```python
from build123d import *

# Parameters (mm, degrees)
SKETCH1_R           = 51.308
BOSS_EXTRUDE1_DEPTH = 92.71
SKETCH2_W           = 103.886
SKETCH2_H           = 103.886
SKETCH2_R           = 1.27
BOSS_EXTRUDE2_DEPTH = 1.27
SHELL1_START        = -92.71
SHELL1_OUTLINE_R    = 50.038
SHELL1_DEPTH        = 92.71
FILLET1_R           = 12.7
SKETCH3_R           = 2.9591
BOSS_EXTRUDE3_DEPTH = 36.83


# Read off the part's stored shape, not the designer's step: Shell1
with BuildPart() as part:
    # Sketch1 → Boss-Extrude1 (new body)
    with BuildSketch(Plane.XY):
        Circle(SKETCH1_R)
    extrude(amount=-BOSS_EXTRUDE1_DEPTH)

    # Sketch2 → Boss-Extrude2 (add)
    with BuildSketch(Plane.XY):
        Rectangle(SKETCH2_W, SKETCH2_H)
        with Locations((43.053, 43.053)):
            Circle(SKETCH2_R, mode=Mode.SUBTRACT)
        with Locations((-43.053, 43.053)):
            Circle(SKETCH2_R, mode=Mode.SUBTRACT)
        with Locations((43.053, -43.053)):
            Circle(SKETCH2_R, mode=Mode.SUBTRACT)
        with Locations((-43.053, -43.053)):
            Circle(SKETCH2_R, mode=Mode.SUBTRACT)
    extrude(amount=-BOSS_EXTRUDE2_DEPTH)

    # Shell1 outline → Shell1 (cut)
    with BuildSketch(Plane.XY.offset(SHELL1_START)):
        Circle(SHELL1_OUTLINE_R)
    extrude(amount=SHELL1_DEPTH, mode=Mode.SUBTRACT)

    # Fillet1
    fillet1_edges = [part.edges().sort_by_distance(p)[0] for p in [
        (51.943, 51.943, -0.635),
        (51.943, -51.943, -0.635),
        (-51.943, -51.943, -0.635),
        (-51.943, 51.943, -0.635),
    ]]
    fillet(fillet1_edges, radius=FILLET1_R)

    # Sketch3 → Boss-Extrude3 (add)
    with BuildSketch(Plane(origin=(0, 0, -1.27), x_dir=(-1, 0, 0), z_dir=(0, 0, -1))):
        with Locations((-43.053, 43.053)):
            Circle(SKETCH3_R)
        with Locations((43.053, 43.053)):
            Circle(SKETCH3_R)
        with Locations((43.053, -43.053)):
            Circle(SKETCH3_R)
        with Locations((-43.053, -43.053)):
            Circle(SKETCH3_R)
    extrude(amount=BOSS_EXTRUDE3_DEPTH)


solid = part.part
```
Check sheet for the modelled part. Datum: model origin and axes. Units: mm. A direction names the side the tool comes from. Give positions to 0.01 mm unless a question says otherwise; leave off trailing zeros. Order: outer loops, then holes, each group sorted by start corner. A loop starts at its lowest first (then second) coordinate and runs counter-clockwise, first axis right, second up. Notation, with made-up numbers: M 9.5,71 L 63.5,71 A24 cw 63.5,88 Z; hole C 43.5,84 d10. An arc over 180 degrees is marked long. Answer in a Markdown table with one row per item.
1) Cross-section at A-A, the plane y = 0. Enter the section's corners in (x, z).
Filled sheet:
| item | result |
|---|---|
| outline | M -51.94,-1.27 L -51.31,-1.27 L -51.31,-92.71 L -50.04,-92.71 L -50.04,0 L -51.94,0 Z; M 50.04,-92.71 L 51.31,-92.71 L 51.31,-1.27 L 51.94,-1.27 L 51.94,0 L 50.04,0 Z |
2) Access from +Z, -Z, +X, -X, +Y, -Y to the whole of each face (thin tool, end or side, straight path). Record for faces 1 (the flat face through (43, -43, -38.1)), 2 (the flat face through (43, 43, -38.1)), 3 (the flat face through (-50.3, -11.3, -1.27)), 4 (the cylindrical face through (48.124, 48.321, -0.644)), 5 (the flat face through (-43, 43, -38.1)).
Filled sheet:
| item | result |
|---|---|
| face 1 | -Z, +X, -Y |
| face 2 | -Z, +X, +Y |
| face 3 | -Z |
| face 4 | +Z, -Z, +X, +Y |
| face 5 | -Z, -X, +Y |
3) Cross-section at C-C, the plane z = -28. Enter the section's corners in (x, y).
Filled sheet:
| item | result |
|---|---|
| outline | C 0,0 d102.62; C -43.05,-43.05 d5.92; C -43.05,43.05 d5.92; C 43.05,-43.05 d5.92; C 43.05,43.05 d5.92; hole C 0,0 d100.08 |
4) Thickness scan on L1, parallel to Y at x = -0.5, z = -28; L2, parallel to Z at x = -31, y = -42; L3, parallel to Y at x = 10.5, z = -42.5. Record the ranges inside material, lowest first. Write a range as [from, to].
Filled sheet:
| item | result |
|---|---|
| L1 | y = [-51.31, -50.04], [50.04, 51.31] |
| L2 | z = [-1.27, 0] |
| L3 | y = [-50.22, -48.92], [48.92, 50.22] |
5) Gauge pin test, flat ends, axial feed: P1, Ø1.8, axis at x = 43.5, y = 42, coming from the -Z side; P2, Ø2, axis at x = -43.053, y = -43.053, coming from the +Z side; P3, Ø6, axis at x = -38.5, y = 31.5, coming from the -Z side; P4, Ø3, axis at x = -14, z = -74.5, coming from the -Y side. Record the tip position at first contact, or that the pin passes through.
Filled sheet:
| item | result |
|---|---|
| P1 | stops at z = -38.1 |
| P2 | stops at z = -1.27 |
| P3 | stops at z = -92.71 |
| P4 | stops at y = -49.76 |
6) Release check for a two-part mould opening along Y. For faces 6 (the flat face through (-43, -43, -38.1)), 7 (the cylindrical face through (-48.321, 48.124, -0.644)), 8 (the cylindrical face through (43.694, 40.164, -19.427)) record: +Y half, -Y half, draft (parallel to the pull), parting line (faces both ways), or undercut.
Filled sheet:
| item | result |
|---|---|
| face 6 | draft |
| face 7 | +Y half |
| face 8 | undercut |
